Could you check a few things on this model? Use its own coordinates, in mm. Round coordinates to 2 decimals unless told otherwise and drop trailing zeros. Loops run counter-clockwise (first coordinate to the right, second up) from the corner with the lowest first, then second, coordinate; pieces in that order, holes last. Notation, with made-up numbers: (89.25, -35) -> (122.25, -35) arc R10 cw to (122.25, -17) -> close; hole circle Ø6 at (85, 65.25). An arc over 180 degrees is marked (long way). Put each result on its own line as item: value. Start each with the question number.
1. Imagine slicing it at D-D, the plane z = -20.3. Please give me the cut outline in (x, y).
2. Imagine slicing it at B-B, the plane x = 0. Please give me the cut outline in (y, z).
3. If we mould it in two halves opening along X, with no side actions, what happens to faces 1 (the cylindrical face through (-29.287, -6.084, -29.248)), 2 (the flat face through (0, -6, 30)), 3 (the cylindrical face through (-1.15, -6.08, -18.08)), 4 (the cylindrical face through (29.248, -6.084, -29.287))? For each: pulls with the +X half, pulls with the -X half, needs draft (parallel to the pull), parting line crosses it, or undercut.
4. Imagine slicing it at C-C, the plane x = -20.3. Please give me the cut outline in (y, z), and give its area (3 significant figures).
5. I need wall thicknesses on line 1 (Z direction, x = 0, y = -3.5); line 2 (X direction, y = -5.75, z = -20.3); line 3 (Z direction, x = -15, y = -11). Which ranges of each line are inside material? Lowest first, please. Write a range as [from, to].
6. Imagine slicing it at A-A, the plane z = 0. Please give me the cut outline in (x, y), and give its area (3 significant figures).
```python
from build123d import *

# Parameters (mm, degrees)
F0_W     = 60
F0_H     = 60
F1_DEPTH = 12
F2_D     = 5
F3_D     = 12
F4_R     = 2.5


with BuildPart() as f1:
    # F0 (on Front) → F1 (new body)
    with BuildSketch(Plane.XZ):
        Rectangle(F0_W, F0_H)
    extrude(amount=F1_DEPTH)

    # F2 (through all)
    with Locations(Plane(origin=(0, 0, 0), x_dir=(1, 0, 0), z_dir=(0, 1, 0))):
        with Locations((0, 20.3), (0, -20.3), (-20.3, 0), (20.3, 0)):
            Hole(F2_D / 2)

    # F3 (through all)
    with Locations(Plane(origin=(0, 0, 0), x_dir=(1, 0, 0), z_dir=(0, 1, 0))):
        with Locations((-20.3, 20.3), (20.3, 20.3), (20.3, -20.3), (-20.3, -20.3)):
            Hole(F3_D / 2)

    # F4
    f4_edges = [f1.edges().sort_by_distance(p)[0] for p in [
        (30, -6, 30),
        (30, -6, -30),
        (-30, -6, -30),
        (-30, -6, 30),
    ]]
    fillet(f4_edges, radius=F4_R)


solid = f1.part
```
Entries:
1. outline: (-30, -12) -> (-26.3, -12) -> (-26.3, 0) -> (-30, 0) -> close; (-14.3, -12) -> (-2.5, -12) -> (-2.5, 0) -> (-14.3, 0) -> close; (2.5, -12) -> (14.3, -12) -> (14.3, 0) -> (2.5, 0) -> close; (26.3, -12) -> (30, -12) -> (30, 0) -> (26.3, 0) -> close
2. outline: (-12, -30) -> (0, -30) -> (0, -22.8) -> (-12, -22.8) -> close; (-12, -17.8) -> (0, -17.8) -> (0, 17.8) -> (-12, 17.8) -> close; (-12, 22.8) -> (0, 22.8) -> (0, 30) -> (-12, 30) -> close
3. face 1: pulls with the -X half
3. face 2: needs draft
3. face 3: undercut
3. face 4: pulls with the +X half
4. outline: (-12, -30) -> (0, -30) -> (0, -26.3) -> (-12, -26.3) -> close; (-12, -14.3) -> (0, -14.3) -> (0, -2.5) -> (-12, -2.5) -> close; (-12, 2.5) -> (0, 2.5) -> (0, 14.3) -> (-12, 14.3) -> close; (-12, 26.3) -> (0, 26.3) -> (0, 30) -> (-12, 30) -> close
4. area: 372 mm^2
5. line 1: [-30, -22.8], [-17.8, 17.8], [22.8, 30]
5. line 2: [-30, -26.3], [-14.3, -2.5], [2.5, 14.3], [26.3, 30]
5. line 3: [-30, -23.11], [-17.49, 17.49], [23.11, 30]
6. outline: (-30, -12) -> (-22.8, -12) -> (-22.8, 0) -> (-30, 0) -> close; (-17.8, -12) -> (17.8, -12) -> (17.8, 0) -> (-17.8, 0) -> close; (22.8, -12) -> (30, -12) -> (30, 0) -> (22.8, 0) -> close
6. area: 600 mm^2
